Input: part model. Units: mm. Frame: model coordinates. A direction names the side the tool comes from. Round coordinates to 2 decimals unless told otherwise and drop trailing zeros. Order: outer loops, then holes, each group sorted by start corner. A loop starts at its lowest first (then second) coordinate and runs counter-clockwise, first axis right, second up.
Item 1: Reachability of faces 4 (the cylindrical face through (7.37, 11.85, -18.43)), 5 (the flat face through (-1, 5, 31.75)), 6 (the cylindrical face through (4.08, 10.22, 22.09)) from +Z, -Z, +X, -X, +Y, -Y: full face, straight path, thin tool, end or side. Return the list, or none.
Item 2: Line query: L1, parallel to X at y = 8.5, z = 22.5; L2, parallel to X at y = 14, z = -14; L3, parallel to X at y = 15.25, z = 18.5. Output: solid intervals per line, ascending.
Item 3: First-contact query: pin 1 (4 mm diameter, centred on x = 1.59, y = 7.94, fed in from +Z); pin 2 (11.5 mm diameter, centred on x = 34.925, z = 0, fed in from +Y) (3 decimals). Flat tips, straight axial feed; report the tip coordinate or a pass-through.
Item 4: Cut plane A-A on z = 0. Output: boundary loops of the cut face in (x, y) (1 decimal).
Item 5: Mould query, pull axis Y, two halves, no side actions, for faces 1 (the flat face through (-1, 0, 0)), 2 (the flat face through (-63.5, 8, 0)), 3 (the cylindrical face through (-55.61, 8.95, 22.09)). Classes: released by +Y, released by -Y, zero draft, split by the parting line, or undercut.
```python
from build123d import *

# Parameters (mm, degrees)
F0_W     = 127
F0_H     = 63.5
F1_DEPTH = 15.875
F3_D     = 6.7564
F3_DEPTH = 19.05
F3_TIP   = 2.0298273432
F5_D     = 9.9314
F7_D     = 5.2324
F7_DEPTH = 7.9375
F7_TIP   = 1.5719715515
F8_R     = 0.79375


with BuildPart() as f1:
    # F0 (on Front) → F1 (new body)
    with BuildSketch(Plane.XZ):
        Rectangle(F0_W, F0_H)
    extrude(amount=-F1_DEPTH)

    # F3
    with Locations(Plane.XY.offset(31.75)):
        with Locations((-52.3875, 7.9375), (1.5875, 7.9375)):
            Hole(F3_D / 2, depth=F3_DEPTH)
            with Locations((0, 0, -(F3_DEPTH + F3_TIP / 2))):  # 118° drill point
                Cone(0, F3_D / 2, F3_TIP, mode=Mode.SUBTRACT)

    # F5 (through all)
    with Locations(Plane.XZ):
        with Locations((34.925, 0)):
            Hole(F5_D / 2)

    # F7
    with Locations(Plane(origin=(0, 15.875, 0), x_dir=(-1, 0, 0), z_dir=(0, 1, 0))):
        with Locations((-7.9375, -15.875)):
            Hole(F7_D / 2, depth=F7_DEPTH)
            with Locations((0, 0, -(F7_DEPTH + F7_TIP / 2))):  # 118° drill point
                Cone(0, F7_D / 2, F7_TIP, mode=Mode.SUBTRACT)

    # F8
    f8_edges = [f1.edges().sort_by_distance(p)[0] for p in [
        (0, 0, 31.75),
        (-63.5, 7.9375, 31.75),
        (0, 15.875, 31.75),
        (63.5, 7.9375, 31.75),
        (63.5, 0, 0),
        (63.5, 15.875, 0),
        (-63.5, 15.875, 0),
        (-63.5, 0, 0),
        (-63.5, 7.9375, -31.75),
        (0, 15.875, -31.75),
        (0, 0, -31.75),
        (63.5, 7.9375, -31.75),
    ]]
    fillet(f8_edges, radius=F8_R)


solid = f1.part
```
From the geometry:
1. face 4: +Y
1. face 5: +Z, +X, -X, +Y, -Y
1. face 6: +Z
2. L1: x = -63.5 to -55.72, -49.06 to -1.74, 4.92 to 63.5
2. L2: x = -63.5 to 6.11, 9.76 to 63.5
2. L3: x = -63.48 to 63.48
3. pin 1: stops at z = 11.87
3. pin 2: stops at y = 15.875
4. outline: (-63.5, 0.8) arc R0.8 ccw to (-62.7, 0) - (30, 0) - (30, 15.9) - (-62.7, 15.9) arc R0.8 ccw to (-63.5, 15.1) - close; (39.9, 0) - (62.7, 0) arc R0.8 ccw to (63.5, 0.8) - (63.5, 15.1) arc R0.8 ccw to (62.7, 15.9) - (39.9, 15.9) - close
5. face 1: released by -Y
5. face 2: zero draft
5. face 3: undercut
